Model file for the job. Use its own axes, mm. Round coordinates to 2 decimals unless told otherwise and drop trailing zeros. Loops run counter-clockwise (first coordinate to the right, second up) from the corner with the lowest first, then second, coordinate; pieces in that order, holes last.
from build123d import *

# Parameters (mm, degrees)
BOSS_EXTRUDE1_DEPTH      = 785
BOSS_EXTRUDE1_DEPTH_BACK = 70
SKETCH3_R                = 10.5
SKETCH3_R_2              = 5
CUT_EXTRUDE1_DEPTH       = 787.986697046


with BuildPart() as part:
    # Sketch1 → Boss-Extrude1 (new, two sides: drawn at the far end of the back side and taken through both)
    with BuildSketch(Plane.XY.offset(-BOSS_EXTRUDE1_DEPTH_BACK)):
        with BuildLine():
            Line((0, 44), (0, 6))
            ThreePointArc((0, 6), (1.757359313, 1.757359313), (6, 0))
            Line((6, 0), (18.96119643, 0))
            ThreePointArc((18.96119643, 0), (23.203837117, 1.757359313), (24.96119643, 6))
            Line((24.96119643, 6), (24.96119643, 44))
            ThreePointArc((24.96119643, 44), (23.203837117, 48.242640687), (18.96119643, 50))
            Line((18.96119643, 50), (6, 50))
            ThreePointArc((6, 50), (1.757359313, 48.242640687), (0, 44))
        make_face()
        with BuildLine():
            Line((3, 44), (3, 6))
            ThreePointArc((3, 6), (3.878679656, 3.878679656), (6, 3))
            Line((6, 3), (18.96119643, 3))
            ThreePointArc((18.96119643, 3), (21.082516774, 3.878679656), (21.96119643, 6))
            Line((21.96119643, 6), (21.96119643, 44))
            ThreePointArc((21.96119643, 44), (21.082516774, 46.121320344), (18.96119643, 47))
            Line((18.96119643, 47), (6, 47))
            ThreePointArc((6, 47), (3.878679656, 46.121320344), (3, 44))
        make_face(mode=Mode.SUBTRACT)
    extrude(amount=BOSS_EXTRUDE1_DEPTH + BOSS_EXTRUDE1_DEPTH_BACK)

    # Sketch3 → Cut-Extrude1 (cut, through all)
    with BuildSketch(Plane(origin=(24.96119643, 0, 0), x_dir=(0, 0, -1), z_dir=(1, 0, 0))):
        with Locations(Location((-17.550291159, 25, 0), (0, 0, 90))):
            Circle(SKETCH3_R)
        with Locations(Location((-62.400291159, 25, 0), (0, 0, 90))):
            Circle(SKETCH3_R_2)
        with BuildLine():
            ThreePointArc((-750, 25), (-760, 35), (-770, 25))
            Line((-770, 25), (-760, 25))
            Line((-760, 25), (-750, 25))
        make_face()
        with BuildLine():
            Line((-760, 25), (-770, 25))
            ThreePointArc((-770, 25), (-760, 15), (-750, 25))
            Line((-750, 25), (-760, 25))
        make_face()
        with Locations(Location((27.299708841, 25, 0), (0, 0, 90))):
            Circle(SKETCH3_R_2)
    extrude(amount=-CUT_EXTRUDE1_DEPTH, mode=Mode.SUBTRACT)


solid = part.part
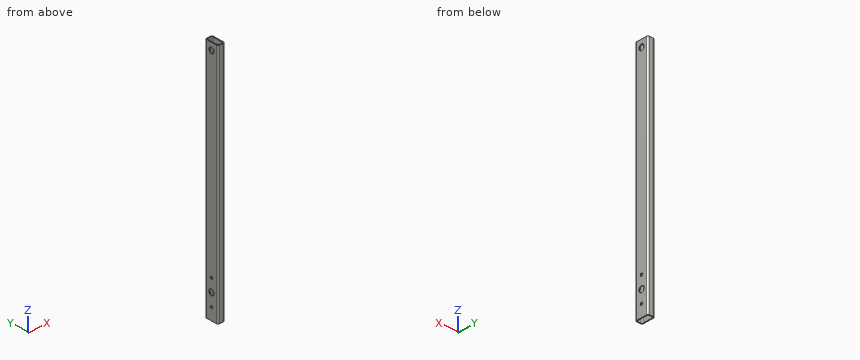
Q1. Slice it at B-B on x = 12.75. Give the cut face in (y, z), plus the area to 3 significant figures.
Q2. Slice it at A-A on z = 760. Give the cut face in (x, y).
Q3. Flat gauge pins, fed straight in: P1, Ø9, axis at y = 25, z = 62.4, coming from the -X side; P2, Ø1, axis at y = 35, z = 360.5, coming from the -X side. Where does each tip first touch, or does it go through?
Q4. Probe line 1 (Z direction, x = 1.75, y = 25); line 2 (Y direction, x = 12, z = 556); line 3 (X direction, y = 42.5, z = 383). List the from-to ranges inside material, lowest first.
Reply:
1. outline: (0, -70) - (3, -70) - (3, 785) - (0, 785) - close; (47, -70) - (50, -70) - (50, 785) - (47, 785) - close
1. area: 5,130 mm2
2. outline: (0, 6) arc R6 ccw to (6, 0) - (18.96, 0) arc R6 ccw to (24.96, 6) - (24.96, 15) - (21.96, 15) - (21.96, 6) arc R3 cw to (18.96, 3) - (6, 3) arc R3 cw to (3, 6) - (3, 15) - (0, 15) - close; (0, 35) - (3, 35) - (3, 44) arc R3 cw to (6, 47) - (18.96, 47) arc R3 cw to (21.96, 44) - (21.96, 35) - (24.96, 35) - (24.96, 44) arc R6 ccw to (18.96, 50) - (6, 50) arc R6 ccw to (0, 44) - close
3. P1: passes through
3. P2: stops at x = 0
4. line 1: z = -70 to -32.3, -22.3 to 7.05, 28.05 to 57.4, 67.4 to 750, 770 to 785
4. line 2: y = 0 to 3, 47 to 50
4. line 3: x = 0 to 3, 21.96 to 24.96
